Here's the drawing with two shaded views (mm, measured from the low corner). I have some questions. Coordinates: 2 decimals unless noted, no trailing zeros. Order: outer loops, then holes, each group sorted by start corner. A loop starts at its lowest first (then second) coordinate and runs counter-clockwise, first axis right, second up. Notation, with made-up numbers: (-6.5, 86.25) - (52.5, 86.25) arc R16 ccw to (52.5, 97.25) - close; hole circle Ø9 at (22, 30.5). An arc over 180 degrees is marked (long way). Answer as a JSON object with one key per item and string values. Group by question number.
(1) Imagine slicing it at B-B, the plane z = 18. Write out the boundary of the cut face in (x, y), and give its area (3 significant figures).
(2) Imagine slicing it at A-A, the plane y = 3.1. Write out the boundary of the cut face in (x, z).
(3) Imagine slicing it at C-C, the plane x = 29. Write out the boundary of the cut face in (y, z), and give its area (3 significant figures).
(4) Please list where these lines run through material, in increasing order: probe 1 along X at (y, z) = (2.85, 22); probe 2 along Z at (x, y) = (27, 2.65); probe 3 along Y at (x, z) = (13.5, 43).
(5) Will this pin go through, and if not, where does the flat tip stop? P1, Ø3, axis at x = 15.5, z = 28, coming from the +Y side.
(6) We'd pull the mould along Z, two halves only. Please class the marked faces 1 and 2: pulls with the +Z half, pulls with the -Z half, needs draft (parallel to the pull), parting line crosses it, or undercut.
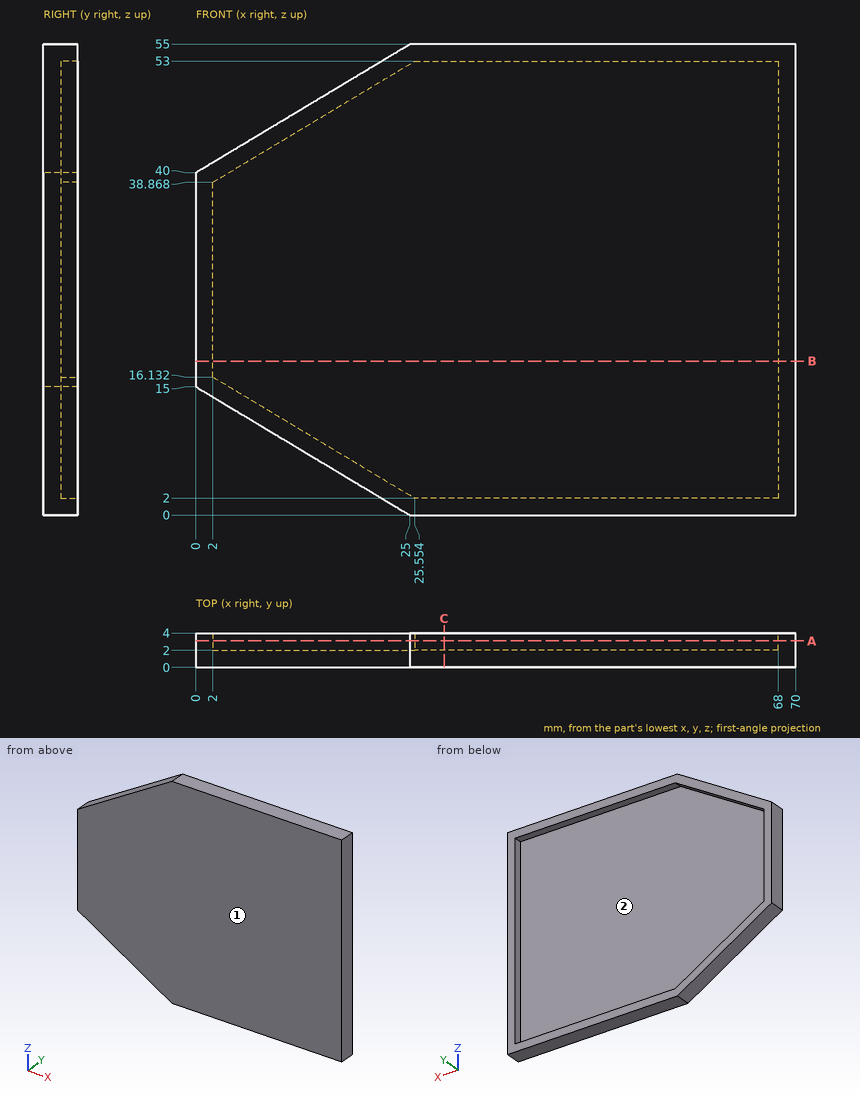
Result set:
{
 "1": {"outline": "(0, 0) - (70, 0) - (70, 4) - (68, 4) - (68, 2) - (2, 2) - (2, 4) - (0, 4) - close", "area": "148 mm^2"},
 "2": {"outline": "(0, 15) - (25, 0) - (70, 0) - (70, 55) - (25, 55) - (0, 40) - close; hole (2, 16.13) - (25.55, 2) - (68, 2) - (68, 53) - (25.55, 53) - (2, 38.87) - close"},
 "3": {"outline": "(0, 0) - (4, 0) - (4, 2) - (2, 2) - (2, 53) - (4, 53) - (4, 55) - (0, 55) - close", "area": "118 mm^2"},
 "4": {"probe 1": "x = 0 to 2, 68 to 70", "probe 2": "z = 0 to 2, 53 to 55", "probe 3": "y = 0 to 2"},
 "5": {"P1": "stops at y = 2"},
 "6": {"face 1": "needs draft", "face 2": "undercut"}
}
